Verification items for the finished model (mm, model axes). A direction names the side the tool comes from. Round coordinates to 2 decimals unless told otherwise and drop trailing zeros. Loops run counter-clockwise (first coordinate to the right, second up) from the corner with the lowest first, then second, coordinate; pieces in that order, holes last. Notation, with made-up numbers: (55.25, -36) -> (71.25, -36) arc R17 ccw to (71.25, -29) -> close; hole circle Ø3 at (84.25, 62). An arc over 180 degrees is marked (long way). Use CSV: the item, a comma, the result in double quotes. Start each with the question number.
```python
from build123d import *

# Parameters (mm, degrees)
ESQUISSE1_R             = 3.15
ESQUISSE1_R_2           = 2
BOSS_EXTRU_1_DEPTH      = 1.6
BOSS_EXTRU_2_START      = -11.5
ESQUISSE2_R             = 9.5
ESQUISSE2_R_2           = 3.15
BOSS_EXTRU_2_DEPTH      = 11.5
CONG_1_R                = 1
BOSS_EXTRU_3_DEPTH      = 13
ESQUISSE4_R             = 2
ENL_V_MAT_EXTRU_1_DEPTH = 40.340310116


with BuildPart() as part:
    # Esquisse1 → Boss.-Extru.1 (new body)
    with BuildSketch(Plane(origin=(0, 0, 0), x_dir=(1, 0, 0), z_dir=(0, 1, 0))):
        with BuildLine():
            Line((0, 11.5), (-25, 11.5))
            ThreePointArc((-25, 11.5), (-31.5, 5), (-25, -1.5))
            Line((-25, -1.5), (-16.90921754, -1.5))
            ThreePointArc((-16.90921754, -1.5), (-13.826301978, -3.956560509), (-15.532463951, -7.510159982))
            Line((-15.532463951, -7.510159982), (-17.532463951, -8.477187494))
            Line((-17.532463951, -8.477187494), (-13, -18.5))
            Line((-13, -18.5), (4.73848504, -10.478394893))
            ThreePointArc((4.73848504, -10.478394893), (11.241697854, 2.423680954), (0, 11.5))
        make_face()
        with Locations(Location((0, 0, 0), (0, 0, 270))):
            Circle(ESQUISSE1_R, mode=Mode.SUBTRACT)
        with Locations(Location((-25, 5, 0), (0, 0, 270))):
            Circle(ESQUISSE1_R_2, mode=Mode.SUBTRACT)
    extrude(amount=BOSS_EXTRU_1_DEPTH)

    # Esquisse2 → Boss.-Extru.2 (add)
    with BuildSketch(Plane(origin=(0, 1.6, 0), x_dir=(1, 0, 0), z_dir=(0, 1, 0)).offset(BOSS_EXTRU_2_START)):
        with Locations(Location((0, 0, 0), (0, 0, 270))):
            Circle(ESQUISSE2_R)
        with Locations(Location((0, 0, 0), (0, 0, 270))):
            Circle(ESQUISSE2_R_2, mode=Mode.SUBTRACT)
    extrude(amount=BOSS_EXTRU_2_DEPTH)

    # Congé1
    cong_1_edges = [part.edges().sort_by_distance(p)[0] for p in [
        (0, -9.9, -9.5),
    ]]
    fillet(cong_1_edges, radius=CONG_1_R)

    # Esquisse3 → Boss.-Extru.3 (add)
    with BuildSketch(Plane(origin=(0, 1.6, 0), x_dir=(1, 0, 0), z_dir=(0, 1, 0))):
        Polygon((-17.532463951, -8.477187494), (-13, -18.5), (-11.633703391, -17.88214048), (-16.182035998, -7.824237002), align=None)
    extrude(amount=BOSS_EXTRU_3_DEPTH)

    # Esquisse4 → Enlèv. mat.-Extru.1 (cut, through all)
    with BuildSketch(Plane.XY):
        with Locations(Location((0, -4, 0), (0, 0, 269.999999976))):
            Circle(ESQUISSE4_R)
    extrude(amount=ENL_V_MAT_EXTRU_1_DEPTH, mode=Mode.SUBTRACT)


solid = part.part
```
Q1. Cross-section at C-C (x = 1.5). State how many separate pieces and enclosed holes the cut face has, and give its area (3 significant figures).
Q2. Release check for a two-part mould opening along X. For faces 1 (the face through (-6, 1.6, 0)), 2 (the face through (-0.766, -5.847, 5.917)), 3 (the face through (0.138, -4.23, -3.147)), 4 (the face through (-13.876, 8.009, 12.924)) record: +X half, -X half, draft (parallel to the pull), parting line (faces both ways), or undercut.
Q3. Cross-section at A-A (x = -26.5). Record the boundary of the cut face in (y, z).
Q4. Depth check by flat-ended pin: pin 1 Ø4.5 at (x, z) = (-25, -5) entering from +Y; pin 2 Ø1.5 at (y, z) = (1, -4) entering from +X; pin 3 Ø9 at (x, z) = (-8.5, 1.5) entering from -Y; pin 4 Ø1.3 at (x, y) = (-22, 1) entering from +Z. Enter the tip coordinate at first touch or a pass-through.
Q5. Tool access check on faces 5 (the face through (-5.78, -4.51, -7.54)), 6 (the face through (-14.4, 14.6, 13.1)). Record the directions out of +Z, -Z, +X, -X, +Y, -Y that give a thin tool (end or side, any length) a straight path to the whole face; none if there is none.
Q6. Thickness scan on L1, parallel to Y at x = 0, z = 6.5; L2, parallel to X at y = -4.5, z = 0; L3, parallel to Y at x = -22.5, z = 0.25. Record the ranges inside material, lowest first. Write a range as from..to.
Q7. Cross-section at B-B (y = 7.75). Record the boundary of the cut face in (x, z).
Q8. Cross-section at D-D (y = -3.25). Record the boundary of the cut face in (x, z), and give its area (3 significant figures).
Answer list:
1,separate pieces,"3"
1,enclosed holes,"0"
1,area,"141 mm2"
2,face 1,"draft"
2,face 2,"undercut"
2,face 3,"undercut"
2,face 4,"+X half"
3,outline,"(0, -11.32) -> (1.6, -11.32) -> (1.6, -6.32) -> (0, -6.32) -> close; (0, -3.68) -> (1.6, -3.68) -> (1.6, 1.32) -> (0, 1.32) -> close"
4,pin 1,"stops at y = 1.6"
4,pin 2,"stops at x = 11.03"
4,pin 3,"stops at y = -9.9"
4,pin 4,"stops at z = 1.5"
5,face 5,"-Y"
5,face 6,"+Z, -Z, +X, -X, +Y"
6,L1,"y = -9.9..-6, -2..1.6"
6,L2,"x = -9.5..-3.15, 3.15..9.5"
6,L3,"y = 0..1.6"
7,outline,"(-17.53, 8.48) -> (-16.18, 7.82) -> (-11.63, 17.88) -> (-13, 18.5) -> close"
8,outline,"(-1.85, 2.55) -> (-1.85, 9.32) arc R9.5 ccw (long way) to (1.85, 9.32) -> (1.85, 2.55) arc R3.15 cw (long way) to start"
8,area,"228 mm2"
